For this review, take the finished solid that the model builds, in its own axes (mm). A direction names the side the tool comes from. Round coordinates to 2 decimals unless told otherwise and drop trailing zeros. Write each loop counter-clockwise with the first axis right and the second up, starting at its lowest first coordinate (ties: lowest second). Pieces come first, ordered by that corner, then holes. Notation, with made-up numbers: M 67.25,76 L 87.25,76 A22 ccw 87.25,109 Z; hole C 51.25,-12.5 d3. An arc over 180 degrees is marked long. Write each question's results on one line, items separated by ' | '. Start each with the question number.
Autodesk Inventor part; units mm, degrees
ref_plane "YZ Plane" through (0, 0, 0) normal (1, 0, 0) x (0, 1, 0)
ref_plane "XZ Plane" through (0, 0, 0) normal (0, 1, 0) x (-1, 0, 0)
ref_plane "XY Plane" through (0, 0, 0) normal (0, 0, 1) x (1, 0, 0)
sketch "Sketch1" plane through (0, 0, 0) normal (1, 0, 0) x (0, 1, 0)
  line L0 (0, 0) -> (0, -25.4)
  line L1 (0, -25.4) -> (25.4, -25.4)
  line L2 (25.4, -25.4) -> (25.4, 0)
  line L3 (25.4, 0) -> (0, 0)
  line L4 (0, 0) -> (0, 2.54)
  line L5 (0, 2.54) -> (25.4, 2.54)
  line L6 (25.4, 2.54) -> (25.4, 0)
  line L7 (0, -25.4) -> (0, -27.94)
  line L8 (0, -27.94) -> (25.4, -27.94)
  line L9 (25.4, -27.94) -> (25.4, -25.4)
  circle A0 centre (13.97, -12.7) radius 7.62
  dimension "d0" = 25.4
  dimension "d1" = 25.4
  dimension "d2" = 2.54
  dimension "d3" = 2.54
ref_plane "Work Plane2" through (2.54, 0, 0) normal (1, 0, 0) x (0, 0, -1)
sketch "Sketch2" plane through (2.54, 0, 0) normal (1, 0, 0) x (0, 0, -1)
  line L0 (27.94, 25.4) -> (-2.54, 25.4)
  line L1 (0, 25.4) -> (0, 0)
  line L2 (-2.54, 25.4) -> (0, 25.4)
  line L3 (-2.54, 25.4) -> (-2.54, 0)
  line L4 (25.4, 0) -> (25.4, 25.4)
  line L5 (27.94, 0) -> (27.94, 25.4)
  line L6 (25.4, 25.4) -> (27.94, 25.4)
  line L7 (27.94, 25.4) -> (27.94, 0)
  line L8 (25.4, 0) -> (25.4, -25.4)
  line L9 (25.4, -25.4) -> (27.94, -25.4)
  line L10 (27.94, -25.4) -> (27.94, 0)
  line L11 (-2.54, 0) -> (-2.54, -25.4)
  line L12 (-2.54, -25.4) -> (0, -25.4)
  line L13 (0, -25.4) -> (0, 0)
  dimension "d10" = 2.54
  dimension "d11" = 25.4
  dimension "d12" = 25.4
extrude "Extrusion2" add sketch "Sketch2" along normal blind 20.32
extrude "Extrusion3" add sketch "Sketch1" along normal blind 2.54
sketch "Sketch3" plane through (2.54, -25.4, 2.54) normal (0, 0, 1) x (1, 0, 0)
  line L0 (0, 0) -> (0, 25.4)
  circle A0 centre (5.08, 15.24) radius 2.54
  circle A1 centre (15.24, 15.24) radius 2.54
  point P0 (-2.54, 25.4)
extrude "Extrusion4" cut sketch "Sketch3" against normal blind 40.3225
fillet "Fillet1" radius 1.5875 1 edges at (22.86, -25.4, 1.27)
fillet "Fillet2" radius 1.5875 1 edges at (22.86, -25.4, -26.67)
fillet "Fillet3" radius 1.5875 1 edges at (22.86, 25.4, 1.27)
fillet "Fillet4" radius 1.5875 1 edges at (22.86, 25.4, -26.67)
fillet "Fillet5" radius 1.5875 2 edges at (2.54, -25.4, 1.27) (2.54, -25.4, -26.67)
fillet "Fillet6" radius 3.81 2 edges at (0, 12.7, -27.94) (0, 12.7, 2.54)
sketch "Sketch4" plane through (2.54, 0, -25.4) normal (0, -1, 0) x (1, 0, 0)
  line L0 (0, 25.4) -> (0, 0)
  line L1 (0, 25.4) -> (0, 0)
  line L2 (0, 0) -> (-2.54, 0)
  line L3 (-2.54, 0) -> (-2.54, 25.4)
  line L4 (-2.54, 25.4) -> (0, 25.4)
extrude "Extrusion5" cut sketch "Sketch4" against normal blind 2.54
sketch "Sketch5" plane through (22.86, -23.8125, -27.94) normal (0, 0, -1) x (-1, 0, 0)
  line L0 (22.86, 26.3525) -> (22.86, 49.2125)
  line L1 (0, 47.625) -> (0, 0)
  line L2 (19.05, 49.2125) -> (19.05, -1.5554)
  circle A0 centre (9.525, 37.7825) radius 2.3812
  point P0 (22.86, 23.8125)
  dimension "d35" = 4.7625
extrude "Extrusion6" cut sketch "Sketch5" against normal blind 38.735
properties part number "Inline Cylinder Mount Bracket" material "Steel, Alloy"
Item 1: We need section B-B on y = -10.16. State the section outline as (x, z) points.
Item 2: For faces 1 (the flat face through (2.54, 8.7, -6.9)), 2 (the cylindrical face through (1.252, 21.238, -14.989)), 3 (the flat face through (2.54, -12, 1)), list the 3-axis set-ups (+Z, -Z, +X, -X, +Y, -Y) from which the entire face can be reached by the end or side of a thin tool; tool diameter is ignored.
Item 3: We need section D-D on z = -14. State the section outline as (x, y) points.
Item 4: For probe 1 along Z at (x, y) = (10.5, -3); probe 2 along Y at (x, z) = (17.78, -27.05); probe 3 along X at (y, z) = (20.5, -3), list the stretches that pass through material, from the lowest coordinate up.
Item 5: We need section A-A on y = -18.5. State the section outline as (x, z) points.
Item 6: Insertion check: P1, Ø0.7, axis at y = -8, z = 1.5, coming from the -X side; P2, Ø6, axis at x = 13.335, y = 13.97, coming from the -Z side; P3, Ø1.2, axis at x = 1.5, z = -27, coming from the -Y side; P4, Ø11.5, axis at y = 16.5, z = -12.5, coming from the +X side. Each pin has a flat end and moves straight along its axis. Give the tip position at first contact, or say it passes through.
Item 7: We need section C-C on x = 17.78. State the section outline as (y, z) points.
Item 8: Mouldability with a two-part tool opening along Z and no side actions: class faces 4 (the flat face through (13, 0, 2.54)), 5 (the flat face through (1, 2.54, -13)), 6 (the flat face through (2, 0, -26)) as pulls with the +Z half, pulls with the -Z half, needs draft (parallel to the pull), parting line crosses it, or undercut.
Numbers:
1) outline: M 2.54,-27.72 A3.81 ccw 3.81,-27.94 L 5.08,-27.94 L 5.08,-25.4 L 2.54,-25.4 Z; M 2.54,0 L 5.08,0 L 5.08,2.54 L 3.81,2.54 A3.81 ccw 2.54,2.32 Z; M 10.16,-27.94 L 15.24,-27.94 L 15.24,-25.4 L 10.16,-25.4 Z; M 10.16,0 L 15.24,0 L 15.24,2.54 L 10.16,2.54 Z; M 20.32,-27.94 L 22.86,-27.94 L 22.86,-25.4 L 20.32,-25.4 Z; M 20.32,0 L 22.86,0 L 22.86,2.54 L 20.32,2.54 Z
2) face 1: +X, +Y, -Y | face 2: +X, -X | face 3: +Z, -Z, -X, -Y
3) outline: M 0,2.54 L 2.54,2.54 L 2.54,6.46 L 0,6.46 Z; M 0,21.48 L 2.54,21.48 L 2.54,25.4 L 0,25.4 Z
4) probe 1: z = -27.94 to -25.4, 0 to 2.54 | probe 2: y = -25.4 to -12.7, -7.62 to 25.4 | probe 3: x = 0 to 2.54
5) outline: M 2.54,-27.72 A3.81 ccw 3.81,-27.94 L 22.86,-27.94 L 22.86,-25.4 L 2.54,-25.4 Z; M 2.54,0 L 22.86,0 L 22.86,2.54 L 3.81,2.54 A3.81 ccw 2.54,2.32 Z
6) P1: stops at x = 2.54 | P2: stops at z = -27.94 | P3: stops at y = 0 | P4: stops at x = 2.54
7) outline: M -25.4,-27.94 L -12.7,-27.94 L -12.7,-25.4 L -25.4,-25.4 Z; M -25.4,0 L -12.7,0 L -12.7,2.54 L -25.4,2.54 Z; M -7.62,-27.94 L 25.4,-27.94 L 25.4,-25.4 L -7.62,-25.4 Z; M -7.62,0 L 25.4,0 L 25.4,2.54 L -7.62,2.54 Z
8) face 4: pulls with the +Z half | face 5: undercut | face 6: needs draft
